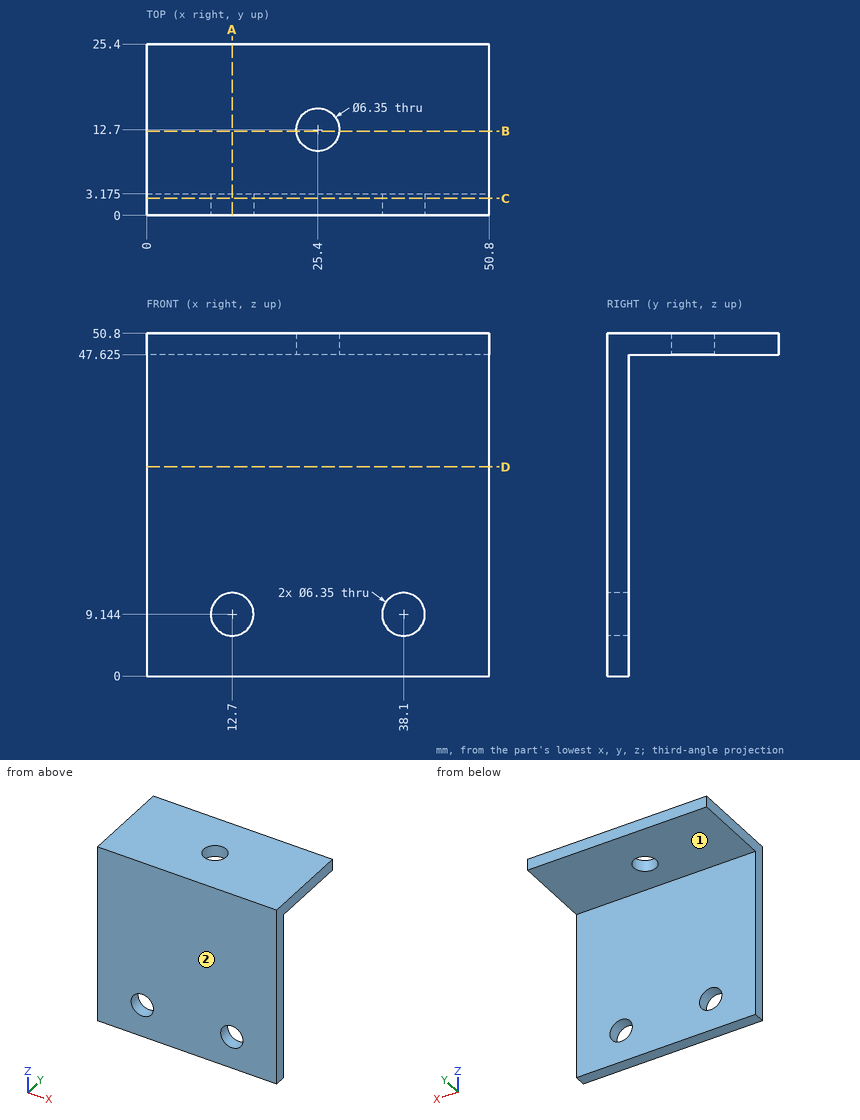
Check sheet for the drawn part. Datum: minimum x, y, z corner. Units: mm. A direction names the side the tool comes from. Round coordinates to 2 decimals unless told otherwise and drop trailing zeros. Write each loop counter-clockwise with the first axis right and the second up, starting at its lowest first coordinate (ties: lowest second). Pieces come first, ordered by that corner, then holes. Notation, with made-up numbers: (-5.5, -19) -> (7.5, -19) arc R32 cw to (7.5, 15) -> close; hole circle Ø1 at (1.5, 74). An arc over 180 degrees is marked (long way). One line per item, written item: value. Start each with the question number.
(1) Cross-section at C-C, the plane y = 2.5. Record the cut outline in (x, z) (3 decimals), and give its area (3 significant figures).
(2) Cross-section at A-A, the plane x = 12.7. Record the cut outline in (y, z) (3 decimals), and give its area (3 significant figures).
(3) Access from +Z, -Z, +X, -X, +Y, -Y to the whole of each face (thin tool, end or side, straight path). Record for the marked faces 1 and 2.
(4) Go/stop test with flat-tipped pins: pin 1 Ø10 at (x, z) = (45, 6.5) entering from +Y (3 decimals); pin 2 Ø6 at (x, y) = (22, 12.5) entering from -Z (3 decimals). Record where each tip stops, or that it passes through.
(5) Cross-section at D-D, the plane z = 31. Record the cut outline in (x, y) (3 decimals), and give its area (3 significant figures).
(6) Cross-section at B-B, the plane y = 12.5. Record the cut outline in (x, z) (3 decimals), and give its area (3 significant figures).
(7) Scan lines: line 1 (Y direction, x = 25.4, z = 49.3) (3 decimals); line 2 (Z direction, x = 38.1, y = 1.75); line 3 (Y direction, x = 38.5, z = 44.5) (3 decimals). Record each from-to range of solid material in increasing order. Write a range as [from, to].
Answer:
1. outline: (0, 0) -> (50.8, 0) -> (50.8, 50.8) -> (0, 50.8) -> close; hole circle Ø6.35 at (12.7, 9.144); hole circle Ø6.35 at (38.1, 9.144)
1. area: 2,520 mm²
2. outline: (0, 0) -> (3.175, 0) -> (3.175, 5.969) -> (0, 5.969) -> close; (0, 12.319) -> (3.175, 12.319) -> (3.175, 47.625) -> (25.4, 47.625) -> (25.4, 50.8) -> (0, 50.8) -> close
2. area: 212 mm²
3. face 1: -Z, +X, -X, +Y
3. face 2: +Z, -Z, +X, -X, -Y
4. pin 1: y = 3.175
4. pin 2: z = 47.625
5. outline: (0, 0) -> (50.8, 0) -> (50.8, 3.175) -> (0, 3.175) -> close
5. area: 161 mm²
6. outline: (0, 47.625) -> (22.231, 47.625) -> (22.231, 50.8) -> (0, 50.8) -> close; (28.569, 47.625) -> (50.8, 47.625) -> (50.8, 50.8) -> (28.569, 50.8) -> close
6. area: 141 mm²
7. line 1: [0, 9.525], [15.875, 25.4]
7. line 2: [0, 5.97], [12.32, 50.8]
7. line 3: [0, 3.175]
